from build123d import *

# Parameters (mm, degrees)
SKETCH1_R           = 2.55
BOSS_EXTRUDE1_DEPTH = 3


with BuildPart() as part:
    # Sketch1 → Boss-Extrude1 (new body)
    with BuildSketch(Plane(origin=(0, 0, 0), x_dir=(1, 0, 0), z_dir=(0, 1, 0))):
        with BuildLine():
            Line((-47, 290), (47, 290))
            ThreePointArc((47, 290), (49.121320344, 289.121320344), (50, 287))
            Line((50, 287), (50, -247))
            ThreePointArc((50, -247), (49.121320344, -249.121320344), (47, -250))
            Line((47, -250), (-47, -250))
            ThreePointArc((-47, -250), (-49.121320344, -249.121320344), (-50, -247))
            Line((-50, -247), (-50, 287))
            ThreePointArc((-50, 287), (-49.121320344, 289.121320344), (-47, 290))
        make_face()
        with Locations((-40, 280)):
            Circle(SKETCH1_R, mode=Mode.SUBTRACT)
        with Locations((0, 280)):
            Circle(SKETCH1_R, mode=Mode.SUBTRACT)
        with Locations((40, 280)):
            Circle(SKETCH1_R, mode=Mode.SUBTRACT)
        with Locations((-40, -240)):
            Circle(SKETCH1_R, mode=Mode.SUBTRACT)
        with Locations((0, -240)):
            Circle(SKETCH1_R, mode=Mode.SUBTRACT)
        with Locations((40, -240)):
            Circle(SKETCH1_R, mode=Mode.SUBTRACT)
        with Locations((-40, 183)):
            Circle(SKETCH1_R, mode=Mode.SUBTRACT)
        with Locations((-40, 70)):
            Circle(SKETCH1_R, mode=Mode.SUBTRACT)
        with Locations((-40, -30)):
            Circle(SKETCH1_R, mode=Mode.SUBTRACT)
        with Locations((-40, -143)):
            Circle(SKETCH1_R, mode=Mode.SUBTRACT)
        with Locations((40, 170)):
            Circle(SKETCH1_R, mode=Mode.SUBTRACT)
        with Locations((40, 70)):
            Circle(SKETCH1_R, mode=Mode.SUBTRACT)
        with Locations((40, -30)):
            Circle(SKETCH1_R, mode=Mode.SUBTRACT)
        with Locations((40, -130)):
            Circle(SKETCH1_R, mode=Mode.SUBTRACT)
        with BuildLine():
            Line((-26.12, 244.57), (-26.12, 264.57))
            ThreePointArc((-26.12, 264.57), (-23.57, 267.12), (-21.02, 264.57))
            Line((-21.02, 264.57), (-21.02, 244.57))
            ThreePointArc((-21.02, 244.57), (-23.57, 242.02), (-26.12, 244.57))
        make_face(mode=Mode.SUBTRACT)
        with BuildLine():
            Line((26.12, 264.57), (26.12, 244.57))
            ThreePointArc((26.12, 244.57), (23.57, 242.02), (21.02, 244.57))
            Line((21.02, 244.57), (21.02, 264.57))
            ThreePointArc((21.02, 264.57), (23.57, 267.12), (26.12, 264.57))
        make_face(mode=Mode.SUBTRACT)
        with BuildLine():
            Line((26.12, 217.43), (26.12, 197.43))
            ThreePointArc((26.12, 197.43), (23.57, 194.88), (21.02, 197.43))
            Line((21.02, 197.43), (21.02, 217.43))
            ThreePointArc((21.02, 217.43), (23.57, 219.98), (26.12, 217.43))
        make_face(mode=Mode.SUBTRACT)
        with BuildLine():
            Line((-21.02, 217.43), (-21.02, 197.43))
            ThreePointArc((-21.02, 197.43), (-23.57, 194.88), (-26.12, 197.43))
            Line((-26.12, 197.43), (-26.12, 217.43))
            ThreePointArc((-26.12, 217.43), (-23.57, 219.98), (-21.02, 217.43))
        make_face(mode=Mode.SUBTRACT)
        with BuildLine():
            Line((-26.12, -177.43), (-26.12, -157.43))
            ThreePointArc((-26.12, -157.43), (-23.57, -154.88), (-21.02, -157.43))
            Line((-21.02, -157.43), (-21.02, -177.43))
            ThreePointArc((-21.02, -177.43), (-23.57, -179.98), (-26.12, -177.43))
        make_face(mode=Mode.SUBTRACT)
        with BuildLine():
            Line((26.12, -157.43), (26.12, -177.43))
            ThreePointArc((26.12, -177.43), (23.57, -179.98), (21.02, -177.43))
            Line((21.02, -177.43), (21.02, -157.43))
            ThreePointArc((21.02, -157.43), (23.57, -154.88), (26.12, -157.43))
        make_face(mode=Mode.SUBTRACT)
        with BuildLine():
            Line((26.12, -204.57), (26.12, -224.57))
            ThreePointArc((26.12, -224.57), (23.57, -227.12), (21.02, -224.57))
            Line((21.02, -224.57), (21.02, -204.57))
            ThreePointArc((21.02, -204.57), (23.57, -202.02), (26.12, -204.57))
        make_face(mode=Mode.SUBTRACT)
        with BuildLine():
            Line((-21.02, -204.57), (-21.02, -224.57))
            ThreePointArc((-21.02, -224.57), (-23.57, -227.12), (-26.12, -224.57))
            Line((-26.12, -224.57), (-26.12, -204.57))
            ThreePointArc((-26.12, -204.57), (-23.57, -202.02), (-21.02, -204.57))
        make_face(mode=Mode.SUBTRACT)
        with BuildLine():
            Line((8, 241), (8, 221))
            ThreePointArc((8, 221), (0, 213), (-8, 221))
            Line((-8, 221), (-8, 241))
            ThreePointArc((-8, 241), (0, 249), (8, 241))
        make_face(mode=Mode.SUBTRACT)
        with BuildLine():
            Line((8, -181), (8, -201))
            ThreePointArc((8, -201), (0, -209), (-8, -201))
            Line((-8, -201), (-8, -181))
            ThreePointArc((-8, -181), (0, -173), (8, -181))
        make_face(mode=Mode.SUBTRACT)
    extrude(amount=BOSS_EXTRUDE1_DEPTH)


solid = part.part
Can you work these out from the model? Positions are in its coordinate system, mm. Give positions to 0.01 mm unless a question says otherwise; leave off trailing zeros. Loops run counter-clockwise (first coordinate to the right, second up) from the corner with the lowest first, then second, coordinate; pieces in that order, holes last. Notation, with made-up numbers: (31, -17) - (76, -17) arc R23 cw to (76, 18) - close; hole circle Ø9 at (28, 36). An arc over 180 degrees is marked (long way). Answer as a JSON object with one key per item and string values.
Q1. Imagine slicing it at B-B on y = 1.1. Give the number of separate pieces and of enclosed holes in the cut face, plus the area to 3 significant figures.
Geometry says:
{"separate pieces": "1", "enclosed holes": "24", "area": "51,700 mm²"}
Q2. Imagine slicing it at A-A on z = -233. Write out the boundary of the cut face in (x, y).
Geometry says:
{"outline": "(-50, 0) - (-8, 0) - (-8, 3) - (-50, 3) - close; (8, 0) - (50, 0) - (50, 3) - (8, 3) - close"}
Q3. If I drill on L1, parallel to X at y = 1.75, z = 30; L2, parallel to X at y = 1, z = 240; L3, parallel to X at y = 2.4, z = 130, over which ranges is the centre line in solid material (lowest first)?
Geometry says:
{"L1": "-50 to -42.55, -37.45 to 37.45, 42.55 to 50", "L2": "-50 to -42.55, -37.45 to -2.55, 2.55 to 37.45, 42.55 to 50", "L3": "-50 to 37.45, 42.55 to 50"}
Q4. Will this pin go through, and if not, where does the flat tip stop? P1, Ø4.5, axis at x = -40, z = 240, coming from the +Y side.
Geometry says:
{"P1": "through"}
